Part model, mm, in its own coordinate system. Face numbers are marked on the shaded views. A direction names the side the tool comes from. Give positions to 0.01 mm unless a question says otherwise; leave off trailing zeros. Write each loop counter-clockwise with the first axis right and the second up, starting at its lowest first coordinate (ties: lowest second). Pieces come first, ordered by that corner, then holes. Notation, with made-up numbers: M -26,73 L -8,73 A21 cw -8,77 Z; hole C -19,46 d1. An arc over 180 degrees is marked long. Use CSV: the item, a comma, the result in double quotes. Start each with the question number.
1. Band-saw the part on D-D, the plane x = 29. List the corners of the cut face in (y, z).
2. 3-axis set-ups, long thin cutter, end or side, ignore diameter. For the marked faces 5, 6 and 7: which of +Z, -Z, +X, -X, +Y, -Y reach the whole face in a straight line?
3. Drill centre lines: line 1 along Y through (x, z) = (-15, 10); line 2 along Y through (x, z) = (-20, 12); line 3 along Y through (x, z) = (-12.5, 23). Where is each one in solid material? Low to high. Write a range as from..to.
4. Band-saw the part on A-A, the plane y = 5.5. List the corners of the cut face in (x, z).
5. Mould opens along X. For the marked faces 1, 2, 3 and 4 say: pulls with the +X half, pulls with the -X half, needs draft (parallel to the pull), parting line crosses it, or undercut.
6. Band-saw the part on C-C, the plane y = -15. List the corners of the cut face in (x, z).
7. Drop flat-ended pins along their axis: pin 1 Ø4 at (x, z) = (7, 24.5) entering from +Y; pin 2 Ø5 at (x, z) = (22, 22.5) entering from +Y; pin 3 Ø10 at (x, y) = (0, -30) entering from -Z; pin 4 Ø22.5 at (x, y) = (-20, 5) entering from -Z. Give the stop position or say it passes through.
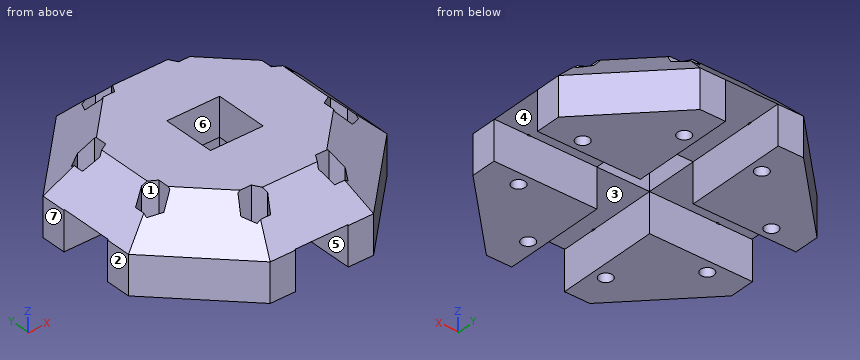
from build123d import *

# Parameters (mm, degrees)
EXTRUDE_1_DEPTH          = 30
CHAMFER_1_SIZE           = 15
SKETCH_2_W               = 15.2
SKETCH_2_H               = 20.4
CUT_EXTRUDE_1_DEPTH      = 50
SKETCH_3_R               = 2.55
CUT_EXTRUDE_2_DEPTH      = 77.811457479
CUT_EXTRUDE_3_DEPTH      = 15
PATTERN_CIRCULAR_1_COUNT = 4
SKETCH_6_W               = 20.4
SKETCH_6_H               = 20.4
CUT_EXTRUDE_4_DEPTH      = 73.325928961


with BuildPart() as part:
    # 스케치1 → 보스-돌출1 (new body)
    with BuildSketch(Plane.XY):
        Polygon((-20, 50), (-50, 20), (-50, -20), (-20, -50), (20, -50), (50, -20), (50, 20), (20, 50), align=None)
    extrude(amount=EXTRUDE_1_DEPTH)

    # 모따기1
    chamfer_1_edges = [part.edges().sort_by_distance(p)[0] for p in [
        (-50, 0, 30),
        (-35, -35, 30),
        (0, -50, 30),
        (35, -35, 30),
        (50, 0, 30),
        (35, 35, 30),
        (0, 50, 30),
        (-35, 35, 30),
    ]]
    chamfer(chamfer_1_edges, length=CHAMFER_1_SIZE)

    # 스케치2 → 컷-돌출1 (cut)
    with BuildSketch(Plane(origin=(50, 0, 0), x_dir=(0, 0, -1), z_dir=(1, 0, 0))):
        with Locations((-7.6, 0)):
            Rectangle(SKETCH_2_W, SKETCH_2_H)
    cut_extrude_1 = extrude(amount=-CUT_EXTRUDE_1_DEPTH, mode=Mode.SUBTRACT)

    # 스케치3 → 컷-돌출2 (cut, through all)
    with BuildSketch(Plane.XY.offset(30)):
        with Locations((36.5, -15)):
            Circle(SKETCH_3_R)
        with Locations((36.5, 15)):
            Circle(SKETCH_3_R)
        with Locations((-15, -36.5)):
            Circle(SKETCH_3_R)
        with Locations((15, -36.5)):
            Circle(SKETCH_3_R)
        with Locations((-36.5, 15)):
            Circle(SKETCH_3_R)
        with Locations((-36.5, -15)):
            Circle(SKETCH_3_R)
        with Locations((15, 36.5)):
            Circle(SKETCH_3_R)
        with Locations((-15, 36.5)):
            Circle(SKETCH_3_R)
    extrude(amount=-CUT_EXTRUDE_2_DEPTH, mode=Mode.SUBTRACT)

    # 스케치4 → 컷-돌출3 (cut)
    with BuildSketch(Plane.XY.offset(30)):
        Polygon((-12.401923789, -32), (-17.598076211, -32), (-20.196152423, -36.5), (-17.598076211, -41), (-12.401923789, -41), (-9.803847577, -36.5), align=None)
        Polygon((32, -12.401923789), (32, -17.598076211), (36.5, -20.196152423), (41, -17.598076211), (41, -12.401923789), (36.5, -9.803847577), align=None)
        Polygon((36.5, 9.803847577), (41, 12.401923789), (41, 17.598076211), (36.5, 20.196152423), (32, 17.598076211), (32, 12.401923789), align=None)
        Polygon((9.803847577, -36.5), (12.401923789, -41), (17.598076211, -41), (20.196152423, -36.5), (17.598076211, -32), (12.401923789, -32), align=None)
        Polygon((-32, 12.401923789), (-32, 17.598076211), (-36.5, 20.196152423), (-41, 17.598076211), (-41, 12.401923789), (-36.5, 9.803847577), align=None)
        Polygon((-36.5, -9.803847577), (-41, -12.401923789), (-41, -17.598076211), (-36.5, -20.196152423), (-32, -17.598076211), (-32, -12.401923789), align=None)
        Polygon((12.401923789, 32), (17.598076211, 32), (20.196152423, 36.5), (17.598076211, 41), (12.401923789, 41), (9.803847577, 36.5), align=None)
        Polygon((-9.803847577, 36.5), (-12.401923789, 41), (-17.598076211, 41), (-20.196152423, 36.5), (-17.598076211, 32), (-12.401923789, 32), align=None)
    extrude(amount=-CUT_EXTRUDE_3_DEPTH, mode=Mode.SUBTRACT)

    # 원형 패턴1: 컷-돌출1 ×4 about axis
    pattern_circular_1_axis = Axis((0, 0, 0), (0, 0, 1))
    for i in range(1, PATTERN_CIRCULAR_1_COUNT):
        add(cut_extrude_1.rotate(pattern_circular_1_axis, i * 360 / PATTERN_CIRCULAR_1_COUNT), mode=Mode.SUBTRACT)

    # 스케치6 → 컷-돌출4 (cut, through all)
    with BuildSketch(Plane(origin=(0, 0, 15.2), x_dir=(-1, 0, 0), z_dir=(0, 0, -1))):
        Rectangle(SKETCH_6_W, SKETCH_6_H)
    extrude(amount=-CUT_EXTRUDE_4_DEPTH, mode=Mode.SUBTRACT)


solid = part.part
Output:
1,outline,"M -41,0 L -10.2,0 L -10.2,15.2 L 10.2,15.2 L 10.2,0 L 41,0 L 41,15 L 19.79,30 L -19.79,30 L -41,15 Z"
2,face 5,"-Z, +Y, -Y"
2,face 6,"+Z, -Z"
2,face 7,"+Z, -Z, -X, +Y, -Y"
3,line 1,"y = -50..-39.05, -33.95..-10.2, 10.2..33.95, 39.05..50"
3,line 2,"y = -50..-10.2, 10.2..50"
3,line 3,"y = -42..-41, -32..32, 41..42"
4,outline,"M -49.8,15.2 L -10.2,15.2 L -10.2,30 L -35,30 Z; M 10.2,15.2 L 49.8,15.2 L 35,30 L 10.2,30 Z"
5,face 1,"undercut"
5,face 2,"pulls with the -X half"
5,face 3,"undercut"
5,face 4,"needs draft"
6,outline,"M -50,0 L -39.05,0 L -39.05,15 L -41,15 L -41,24 L -50,15 Z; M -33.95,0 L -10.2,0 L -10.2,15.2 L 10.2,15.2 L 10.2,0 L 33.95,0 L 33.95,15 L 32,15 L 32,30 L -32,30 L -32,15 L -33.95,15 Z; M 39.05,0 L 50,0 L 50,15 L 41,24 L 41,15 L 39.05,15 Z"
7,pin 1,"stops at y = 42.5"
7,pin 2,"stops at y = 41.72"
7,pin 3,"stops at z = 15.2"
7,pin 4,"stops at z = 0"
